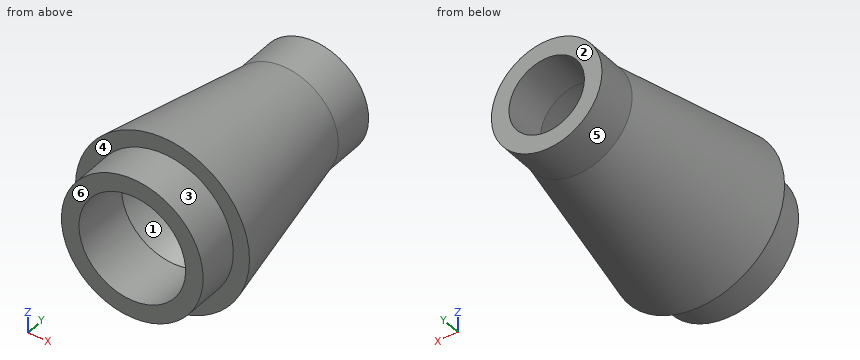
```python
from build123d import *

# Parameters (mm, degrees)
SHELL1_T = -0.7874


with BuildPart() as part:
    # Sketch1 → Revolve1 (revolve)
    with BuildSketch(Plane.XY, mode=Mode.PRIVATE) as revolve1_sk:
        Polygon((0, 11.43), (-2.4765, 11.43), (-2.4765, 9.525), (-3.8989, 1.905), (-3.175, 1.905), (-3.175, 0), (0, 0), align=None)
    revolve(revolve1_sk.sketch.rotate(Axis((0, 0, 0), (0, 1, 0)), 270), axis=Axis((0, 0, 0), (0, 1, 0)))

    # Shell1
    shell1_openings = [part.faces().sort_by_distance(p)[0] for p in [
        (0, 0, 0),
        (0, 11.43, 0),
    ]]
    offset(amount=SHELL1_T, openings=shell1_openings, kind=Kind.INTERSECTION)


solid = part.part
```
Can you work these out from the model? Positions are in its coordinate system, mm. Face numbers are marked on the shaded views. A direction names the side the tool comes from. Round coordinates to 2 decimals unless told otherwise and drop trailing zeros. Order: outer loops, then holes, each group sorted by start corner. A loop starts at its lowest first (then second) coordinate and runs counter-clockwise, first axis right, second up.
(1) On a 3-axis mill with a long thin cutter (end or side, diameter ignored), from which of +Z, -Z, +X, -X, +Y, -Y can I reach the whole of each face in a straight line? I mean the marked faces 4, 5 and 6. Say none if no direction works.
Results are:
face 4: -Y
face 5: +Y
face 6: +Z, -Z, +X, -X, -Y
(2) We'd pull the mould along X, two halves only. Please class the marked faces 1, 2 and 3: +X half, -X half, draft (parallel to the pull), parting line (faces both ways), or undercut.
Results are:
face 1: undercut
face 2: draft
face 3: parting line
(3) I'm going to push flat-ended pins straight in: pin 1 (3 mm diameter, centred on x = 0, z = 0, fed in from -Y) (3 decimals); pin 2 (4 mm diameter, centred on y = 8, z = 0, fed in from -X); pin 3 (2 mm diameter, centred on x = -0.5, y = 7, fed in from -Z); pin 4 (1.5 mm diameter, centred on x = 1, y = 7.5, fed in from +Z). Where does each tip first touch, or does it pass through?
Results are:
pin 1: passes through
pin 2: stops at x = -3.13
pin 3: stops at z = -3.12
pin 4: stops at z = 2.92
(4) If I drill on L1, parallel to X at y = 0.9, z = 0 (3 decimals); L2, parallel to X at y = 10.5, z = 0; L3, parallel to Z at x = 0.25, y = 3.75, over which ranges is the centre line in solid material (lowest first)?
Results are:
L1: x = -3.175 to -2.388, 2.388 to 3.175
L2: x = -2.48 to -1.69, 1.69 to 2.48
L3: z = -3.55 to -2.74, 2.74 to 3.55
(5) If we section it at B-B (y = 8): Please give me the cut outline in (x, z), plus the area to 3 significant figures.
Results are:
outline: circle Ø5.52 at (0, 0); hole circle Ø3.92 at (0, 0)
area: 11.9 mm2
(6) If we section it at A-A (z = 0): Please give me the cut outline in (x, y) (1 decimal), plus the area to 3 significant figures.
Results are:
outline: (-3.9, 1.9) - (-3.2, 1.9) - (-3.2, 0) - (-2.4, 0) - (-2.4, 2.7) - (-3, 2.7) - (-1.7, 9.5) - (-1.7, 11.4) - (-2.5, 11.4) - (-2.5, 9.5) - close; (1.7, 9.5) - (3, 2.7) - (2.4, 2.7) - (2.4, 0) - (3.2, 0) - (3.2, 1.9) - (3.9, 1.9) - (2.5, 9.5) - (2.5, 11.4) - (1.7, 11.4) - close
area: 19.2 mm2
(7) If we section it at C-C (y = 6.5): Please give me the cut outline in (x, z), plus the area to 3 significant figures.
Results are:
outline: circle Ø6.08 at (0, 0); hole circle Ø4.48 at (0, 0)
area: 13.3 mm2
